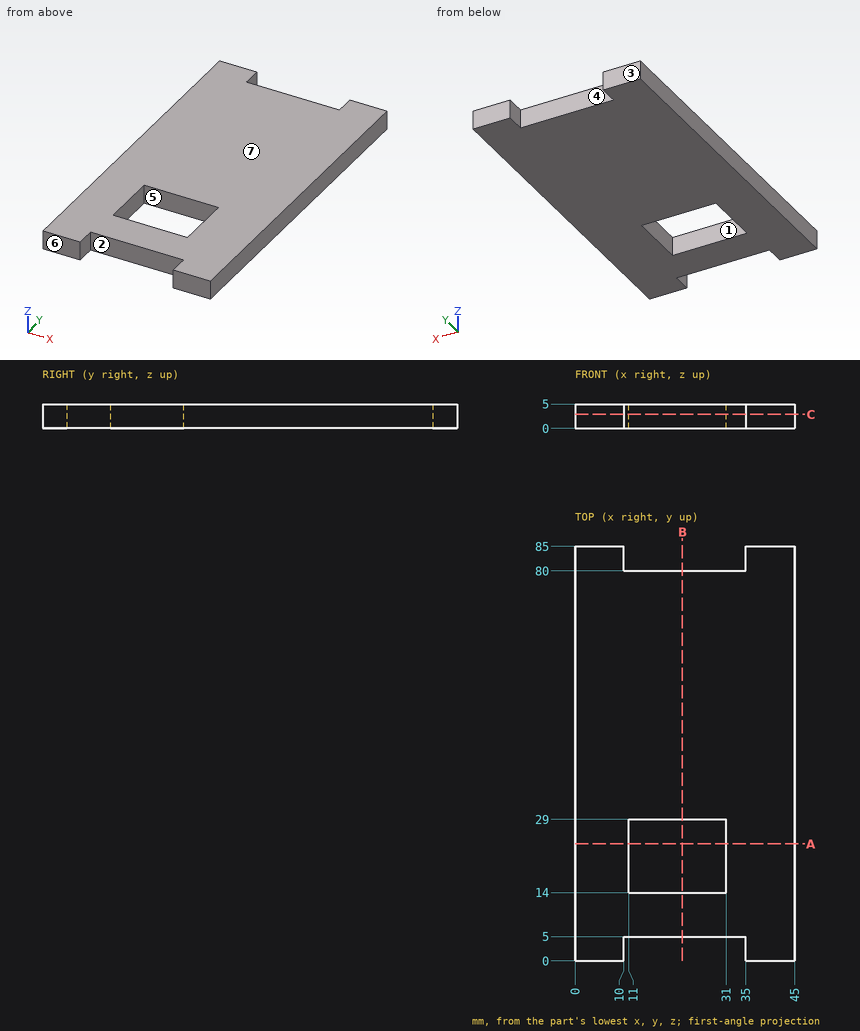
Here's the drawing with two shaded views (mm, measured from the low corner). I have some questions. A direction names the side the tool comes from. Give positions to 0.01 mm unless a question says otherwise; leave off trailing zeros. Loops run counter-clockwise (first coordinate to the right, second up) from the corner with the lowest first, then second, coordinate; pieces in that order, holes last. Notation, with made-up numbers: (80, -4.75) - (102, -4.75) arc R4 ccw to (102, 1.25) - close; hole circle Ø10 at (77, -8.5). An arc over 180 degrees is marked (long way). Answer in a Markdown table with one row per item. Add a question column.
Q1. We'd pull the mould along Y, two halves only. Please class the marked faces 4, 5, 6 and 7: +Y half, -Y half, draft (parallel to the pull), parting line (faces both ways), or undercut.
Q2. If we section it at C-C (z = 2.85): List the corners of the cut face in (x, y) for me.
Q3. If we section it at A-A (y = 24): List the corners of the cut face in (x, z) for me, plus the area to 3 significant figures.
Q4. Which directions (+Z, -Z, +X, -X, +Y, -Y) give clear straight access to the entire face, cutting with the end or side of a thin tool? Please do the marked faces 1, 2 and 3.
Q5. For pin 1 (2.5 mm diameter, centred on y = 2.5, z = 2.5, fed in from -X); pin 2 (2.5 mm diameter, centred on x = 26.5, z = 3.5, fed in from +Y), each with a flat end and sliding along its axis, tell me the tip position at first contact or that it passes through.
Q6. Please list where these lines run through material, in increasing order: L1, parallel to X at y = 27.5, z = 3.5; L2, parallel to X at y = 81, z = 4.75; L3, parallel to Y at x = 24, z = 2.7. Write a range as from..to.
Q7. If we section it at B-B (x = 22): List the corners of the cut face in (y, z) for me.
The answers:
| question | item | result |
|---|---|---|
| 1 | face 4 | +Y half |
| 1 | face 5 | undercut |
| 1 | face 6 | -Y half |
| 1 | face 7 | draft |
| 2 | outline | (0, 0) - (10, 0) - (10, 5) - (35, 5) - (35, 0) - (45, 0) - (45, 85) - (35, 85) - (35, 80) - (10, 80) - (10, 85) - (0, 85) - close; hole (11, 14) - (31, 14) - (31, 29) - (11, 29) - close |
| 3 | outline | (0, 0) - (11, 0) - (11, 5) - (0, 5) - close; (31, 0) - (45, 0) - (45, 5) - (31, 5) - close |
| 3 | area | 125 mm^2 |
| 4 | face 1 | +Z, -Z |
| 4 | face 2 | +Z, -Z, -Y |
| 4 | face 3 | +Z, -Z, +X, -X, +Y |
| 5 | pin 1 | stops at x = 0 |
| 5 | pin 2 | stops at y = 80 |
| 6 | L1 | x = 0..11, 31..45 |
| 6 | L2 | x = 0..10, 35..45 |
| 6 | L3 | y = 5..14, 29..80 |
| 7 | outline | (5, 0) - (14, 0) - (14, 5) - (5, 5) - close; (29, 0) - (80, 0) - (80, 5) - (29, 5) - close |
